Build history of the part. All positions in model axes, mm. A direction names the side the tool comes from. Give positions to 0.01 mm unless a question says otherwise; leave off trailing zeros. Write each loop counter-clockwise with the first axis right and the second up, starting at its lowest first coordinate (ties: lowest second). Pieces come first, ordered by that corner, then holes. Notation, with made-up numbers: M 86.25,-40 L 110.25,-40 A29 cw 110.25,-18 Z; hole C 68.5,36 d11. An arc over 180 degrees is marked long. Return JSON: item names as keys, results as strings. Group by question number.
Q1. Band-saw the part on C-C, the plane z = 5.5. Give the cut face in (x, y), then the cut area to 3 significant figures.
Q2. Pull direction Y, two halves, no side cores. Call faces 1 (the flat face through (8, 0, 0)), 2 (the cylindrical face through (8.767, 16.856, 3.704)), 3 (the flat face through (0, 16, 5)): +Y half, -Y half, draft (parallel to the pull), parting line (faces both ways), or undercut.
Q3. Band-saw the part on A-A, the plane x = 0. Give the cut face in (y, z), then the cut area to 3 significant figures.
Q4. Tool access for faces 4 (the cylindrical face through (15.5, -4.88, 6.48)), 5 (the flat face through (-4, 16, 8)): list every direction of +Z, -Z, +X, -X, +Y, -Y with a clear straight run to the whole face (end or side of a thin tool).
Q5. Flat gauge pins, fed straight in: pin 1 Ø3 at (x, z) = (13, 4) entering from -Y; pin 2 Ø4 at (x, z) = (-12, 3) entering from +Y; pin 3 Ø16 at (x, y) = (-0.5, -4.5) entering from +Z; pin 4 Ø10 at (x, y) = (0, 0) entering from +Z. Where does each tip first touch, or does it go through?
Q6. Wall check: probe 1 along Y at (x, z) = (0, 6.1); probe 2 along Y at (x, z) = (0, 3.6); probe 3 along Z at (x, y) = (-6, 6). Give the ranges that are in metal, low to high.
Autodesk Fusion 360 part; units mm, degrees
sketch "Sketch1" plane through (0, 0, 0) normal (0, 0, 1) x (1, 0, 0)
  circle A0 centre (0, 0) radius 16.25
  circle A1 centre (0, 0) radius 19
  circle A2 centre (0, 0) radius 6.4
  dimension "d1" = 32.5
  dimension "d2" = 38
  dimension "d3" = 12.8
extrude "Extrude1" add sketch "Sketch1" along normal blind 8 contours A1
extrude "Extrude2" add sketch "Sketch1" along normal blind 3 contours A0
chamfer "Chamfer1" distance 1 angle 45 1 edges at (-17.7142, -6.8707, 8)
chamfer "Chamfer2" distance 1 angle 45 1 edges at (-5.9669, 2.3143, 0)
sketch "Sketch2" plane through (0, 0, 3) normal (0, 0, 1) x (-1, 0, 0)
  circle A0 centre (0, 0) radius 6.4
  circle A1 centre (0, 0) radius 16.25
  circle A2 centre (0, 0) radius 15
  dimension "d10" = 30
extrude "Extrude3" add sketch "Sketch2" along normal blind 2 contours A1
fillet "Fillet1" radius 0.5 1 edges at (13.9849, -5.4242, 5)
chamfer "Chamfer3" distance 0.5 angle 45 1 edges at (-17.7142, -6.8707, 0)
From the geometry:
{
 "1": {"outline": "C 0,0 d38; hole C 0,0 d32.5", "area": "305 mm^2"},
 "2": {"face 1": "draft", "face 2": "parting line", "face 3": "undercut"},
 "3": {"outline": "M -19,0.5 L -18.5,0 L -7.4,0 L -6.4,1 L -6.4,3 L -15,3 L -15,4.5 A0.5 ccw -15.5,5 L -16.25,5 L -16.25,8 L -18,8 L -19,7 Z; M 6.4,1 L 7.4,0 L 18.5,0 L 19,0.5 L 19,7 L 18,8 L 16.25,8 L 16.25,5 L 15.5,5 A0.5 ccw 15,4.5 L 15,3 L 6.4,3 Z", "area": "106 mm^2"},
 "4": {"face 4": "+Z", "face 5": "+Z, +X, -X, +Y, -Y"},
 "5": {"pin 1": "stops at y = -15.12", "pin 2": "stops at y = 16.16", "pin 3": "stops at z = 3", "pin 4": "passes through"},
 "6": {"probe 1": "y = -19 to -16.25, 16.25 to 19", "probe 2": "y = -19 to -15, 15 to 19", "probe 3": "z = 0 to 3"}
}
